Can you work these out from the drawing? Everything is in mm from the part's minimum corner. Give positions to 0.01 mm unless a question says otherwise; leave off trailing zeros. Order: outer loops, then holes, each group sorted by start corner. A loop starts at its lowest first (then second) coordinate and runs counter-clockwise, first axis right, second up. Notation, with made-up numbers: M 4,60.25 L 47,60.25 A27 cw 47,90.25 Z; hole C 8.25,50.5 d3. An arc over 180 degrees is marked long. Use a Markdown table: item, result. Add a question column.
Item 1: Suppose I cut it at D-D on z = 54.5. Write out the boundary of the cut face in (x, y), plus the area to 3 significant figures.
Item 2: Suppose I cut it at A-A on x = 12. Write out the boundary of the cut face in (y, z).
Item 3: Suppose I cut it at C-C on z = 12. Write out the boundary of the cut face in (x, y), plus the area to 3 significant figures.
Item 4: If I drill on L1, parallel to X at y = 3.3, z = 12; L2, parallel to X at y = 1.55, z = 8.5; L3, parallel to Z at x = 17, y = 1.6, over which ranges is the centre line in solid material (lowest first)? Write a range as from..to.
Item 5: I'm going to push a flat-ended pin straight in: pin 1 Ø2 at (x, z) = (19.5, 42.5) entering from -Y. Where does the tip first touch, or does it pass through?
Item 6: If we mould it in two halves opening along X, with no side actions, what happens to the marked faces 1 and 2? For each: released by +X, released by -X, zero draft, split by the parting line, or undercut.
Item 7: Suppose I cut it at B-B on y = 2.5. Write out the boundary of the cut face in (x, z), plus the area to 3 significant figures.
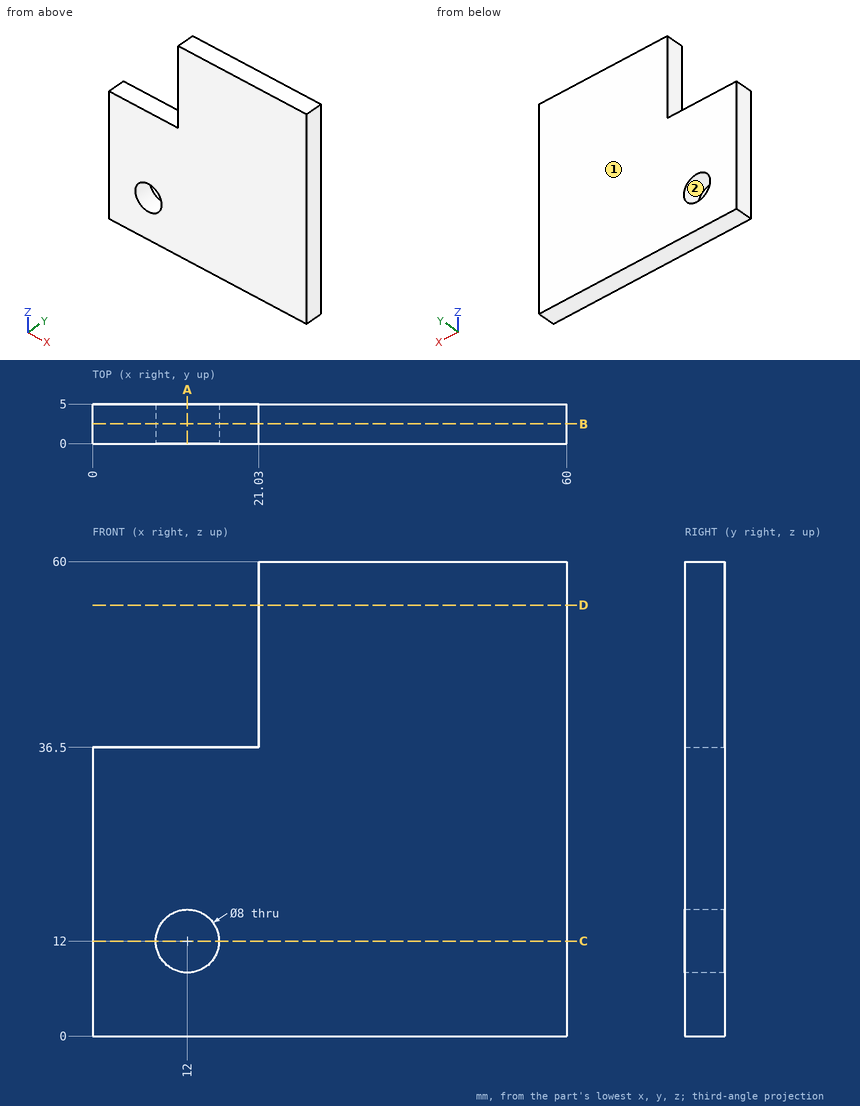
Findings below:
| question | item | result |
|---|---|---|
| 1 | outline | M 21.03,0 L 60,0 L 60,5 L 21.03,5 Z |
| 1 | area | 195 mm^2 |
| 2 | outline | M 0,0 L 5,0 L 5,8 L 0,8 Z; M 0,16 L 5,16 L 5,36.5 L 0,36.5 Z |
| 3 | outline | M 0,0 L 8,0 L 8,5 L 0,5 Z; M 16,0 L 60,0 L 60,5 L 16,5 Z |
| 3 | area | 260 mm^2 |
| 4 | L1 | x = 0..8, 16..60 |
| 4 | L2 | x = 0..10.06, 13.94..60 |
| 4 | L3 | z = 0..36.5 |
| 5 | pin 1 | passes through |
| 6 | face 1 | zero draft |
| 6 | face 2 | undercut |
| 7 | outline | M 0,0 L 60,0 L 60,60 L 21.03,60 L 21.03,36.5 L 0,36.5 Z; hole C 12,12 d8 |
| 7 | area | 3,060 mm^2 |
